Input: part model. Units: mm. Frame: model coordinates. A direction names the side the tool comes from. Give positions to 0.01 mm unless a question says otherwise; leave off trailing zeros. Loops run counter-clockwise (first coordinate to the right, second up) from the corner with the lowest first, then second, coordinate; pieces in that order, holes last. Notation, with made-up numbers: M -27.5,-17.5 L 13.5,-17.5 A34 ccw 13.5,14.5 Z; hole C -32.75,-33.75 d8. An arc over 180 degrees is marked long. One line per item, written item: value. Start each with the question number.
(1) Section A-A on z = 53.15. Output: boundary loops of the cut face in (x, y), plus the area to 3 significant figures.
(2) Pull-direction query (Y, two-part tool) for faces 1 (the cylindrical face through (-9.764, 74.362, 6.409)), 2 (the flat face through (-42.6, 3, 20)), 3 (the flat face through (-48, 3, 64.95)); classes: released by +Y, released by -Y, zero draft, split by the parting line, or undercut.
(3) Access query for faces 4 (the flat face through (-50, 32.697, 20)), 5 (the flat face through (-42.6, 3, 69)), 6 (the flat face through (-24, -8, 10)). Directions: +Z, -Z, +X, -X, +Y, -Y. A direction counts if a zero-diameter tool reaches every point of the face in a straight line with its end or side. Return the directions, or none.
(4) Pin query (flat end, axial travel): P1, Ø3, axis at y = -5.37, z = 67.95, coming from the -X side; P2, Ø1.5, axis at x = -36.5, y = 32, coming from the +Z side; P3, Ø10.5, axis at x = -52, z = 23, coming from the +Y side. Return the tip coordinate at first contact, or that it passes through.
(5) Section B-B on x = 0. Output: boundary loops of the cut face in (y, z).
(6) Section C-C on z = 38. Output: boundary loops of the cut face in (x, y), plus the area to 3 significant figures.
(7) Ray query, line 1 along Y through (x, z) = (-46.8, 67.95); line 2 along X through (y, z) = (28.5, 33); line 3 along Y through (x, z) = (-43, 18). Return the intervals inside material, ascending. Write a range as from..to.
```python
from build123d import *

# Parameters (mm, degrees)
SKETCH1_R           = 75
BASE_PLATE_DEPTH    = 15
SKETCH2_R           = 4.5
DRIVE_HOLES_DEPTH   = 10
CHAMFER1_SIZE       = 1
BASE_START          = 45
BASE_FIN_DEPTH      = 5
BASE_START_2        = 85
BASE_FIN_2_DEPTH    = 5
CUT_EXTRUDE1_REACH  = 122
CUT_EXTRUDE2_REACH  = 122
SKETCH7_R           = 1.75
BOSS_EXTRUDE1_DEPTH = 5.6
SKETCH9_R           = 1.75
CUT_EXTRUDE3_DEPTH  = 5.6
SKETCH10_W          = 4.6
SKETCH10_H          = 2.5
SKETCH10_W_2        = 6
CUT_EXTRUDE4_DEPTH  = 5.6
CUT_EXTRUDE5_DEPTH  = 2.6
BOSS_EXTRUDE2_DEPTH = 1.38
FILLET1_R           = 2
FILLET2_R           = 2
CUT_EXTRUDE6_REACH  = 37
SKETCH13_R          = 12.7
BOSS_EXTRUDE4_START = 20
BOSS_EXTRUDE4_DEPTH = 2.5
BOSS_EXTRUDE5_START = 20
BOSS_EXTRUDE5_DEPTH = 2.5
FILLET4_R           = 2


with BuildPart() as part:
    # Sketch1 → Base Plate (new body)
    with BuildSketch(Plane.XY):
        Circle(SKETCH1_R)
    extrude(amount=BASE_PLATE_DEPTH)

    # Sketch2 → Drive Holes (cut)
    with BuildSketch(Plane(origin=(0, 0, 0), x_dir=(-1, 0, 0), z_dir=(0, 0, -1))):
        with Locations((0, -25)):
            Circle(SKETCH2_R)
        with Locations((-23.776412907, -7.725424859)):
            Circle(SKETCH2_R)
        with Locations((-14.694631307, 20.225424859)):
            Circle(SKETCH2_R)
        with Locations((14.694631307, 20.225424859)):
            Circle(SKETCH2_R)
        with Locations((23.776412907, -7.725424859)):
            Circle(SKETCH2_R)
    extrude(amount=-DRIVE_HOLES_DEPTH, mode=Mode.SUBTRACT)

    # Chamfer1
    chamfer1_edges = [part.edges().sort_by_distance(p)[0] for p in [
        (28.276412907, -7.725424859, 0),
        (19.194631307, 20.225424859, 0),
        (-10.194631307, 20.225424859, 0),
        (-19.276412907, -7.725424859, 0),
        (4.5, -25, 0),
    ]]
    chamfer(chamfer1_edges, length=CHAMFER1_SIZE)

    # Sketch4 → Base Fin (add)
    with BuildSketch(Plane(origin=(0, 0, 0), x_dir=(0, 0, -1), z_dir=(1, 0, 0)).offset(BASE_START)):
        with BuildLine():
            Line((-15, 50), (-65.791986374, 16.233382914))
            ThreePointArc((-65.791986374, 16.233382914), (-74.493324261, 0), (-65.791986374, -16.233382914))
            Line((-65.791986374, -16.233382914), (-15, -50))
            Line((-15, -50), (-15, 50))
        make_face()
    extrude(amount=-BASE_FIN_DEPTH)

    # Sketch5 → Base Fin 2 (add)
    with BuildSketch(Plane.ZY.offset(-40).offset(BASE_START_2)):
        with BuildLine():
            Line((15, 50), (15, -50))
            Line((15, -50), (65.791986374, -16.233382914))
            ThreePointArc((65.791986374, -16.233382914), (74.493324261, 0), (65.791986374, 16.233382914))
            Line((65.791986374, 16.233382914), (15, 50))
        make_face()
    extrude(amount=-BASE_FIN_2_DEPTH)

    # Sketch6 → Cut-Extrude1 (cut, up to next)
    with BuildSketch(Plane.ZY.offset(45), mode=Mode.PRIVATE) as cut_extrude1_sk1:
        with BuildLine():
            Line((64, 8.832406236), (64, -9.567593764))
            ThreePointArc((64, -9.567593764), (63.487436867, -10.805030631), (62.25, -11.317593764))
            Line((62.25, -11.317593764), (24.05, -11.317593764))
            ThreePointArc((24.05, -11.317593764), (22.812563133, -10.805030631), (22.3, -9.567593764))
            Line((22.3, -9.567593764), (22.3, 8.832406236))
            ThreePointArc((22.3, 8.832406236), (22.812563133, 10.069843103), (24.05, 10.582406236))
            Line((24.05, 10.582406236), (62.25, 10.582406236))
            ThreePointArc((62.25, 10.582406236), (63.487436867, 10.069843103), (64, 8.832406236))
        make_face()
    cut_extrude1_tool1 = extrude(cut_extrude1_sk1.sketch, amount=-CUT_EXTRUDE1_REACH, mode=Mode.PRIVATE) & part.part
    add(cut_extrude1_tool1.solids().sort_by_distance((-45, -0.367594, 43.15))[0], mode=Mode.SUBTRACT)

    # Sketch7 → Cut-Extrude2 (cut, up to next)
    with BuildSketch(Plane.ZY.offset(45), mode=Mode.PRIVATE) as cut_extrude2_sk1:
        with Locations((18.35, 4.632406236)):
            Circle(SKETCH7_R)
    cut_extrude2_tool1 = extrude(cut_extrude2_sk1.sketch, amount=-CUT_EXTRUDE2_REACH, mode=Mode.PRIVATE) & part.part
    add(cut_extrude2_tool1.solids().sort_by_distance((-45, 4.632406, 18.35))[0], mode=Mode.SUBTRACT)
    # Sketch7 → Cut-Extrude2 (cut, up to next)
    with BuildSketch(Plane.ZY.offset(45), mode=Mode.PRIVATE) as cut_extrude2_sk2:
        with Locations((18.35, -5.367593764)):
            Circle(SKETCH7_R)
    cut_extrude2_tool2 = extrude(cut_extrude2_sk2.sketch, amount=-CUT_EXTRUDE2_REACH, mode=Mode.PRIVATE) & part.part
    add(cut_extrude2_tool2.solids().sort_by_distance((-45, -5.367594, 18.35))[0], mode=Mode.SUBTRACT)
    # Sketch7 → Cut-Extrude2 (cut, up to next)
    with BuildSketch(Plane.ZY.offset(45), mode=Mode.PRIVATE) as cut_extrude2_sk3:
        with Locations((67.95, -5.367593764)):
            Circle(SKETCH7_R)
    cut_extrude2_tool3 = extrude(cut_extrude2_sk3.sketch, amount=-CUT_EXTRUDE2_REACH, mode=Mode.PRIVATE) & part.part
    add(cut_extrude2_tool3.solids().sort_by_distance((-45, -5.367594, 67.95))[0], mode=Mode.SUBTRACT)
    # Sketch7 → Cut-Extrude2 (cut, up to next)
    with BuildSketch(Plane.ZY.offset(45), mode=Mode.PRIVATE) as cut_extrude2_sk4:
        with Locations((67.95, 4.632406236)):
            Circle(SKETCH7_R)
    cut_extrude2_tool4 = extrude(cut_extrude2_sk4.sketch, amount=-CUT_EXTRUDE2_REACH, mode=Mode.PRIVATE) & part.part
    add(cut_extrude2_tool4.solids().sort_by_distance((-45, 4.632406, 67.95))[0], mode=Mode.SUBTRACT)

    # Sketch8 → Boss-Extrude1 (add)
    with BuildSketch(Plane.ZY.offset(45)):
        with BuildLine():
            Line((70.95, 4.632406236), (70.95, -5.367593764))
            ThreePointArc((70.95, -5.367593764), (67.95, -8.367593764), (64.95, -5.367593764))
            Line((64.95, -5.367593764), (64.95, 4.632406236))
            ThreePointArc((64.95, 4.632406236), (67.95, 7.632406236), (70.95, 4.632406236))
        make_face()
        with BuildLine():
            Line((15, 7.632406236), (15, 0))
            Line((15, 0), (15, -8.367593764))
            Line((15, -8.367593764), (18.35, -8.367593764))
            ThreePointArc((18.35, -8.367593764), (20.471320344, -7.488914107), (21.35, -5.367593764))
            Line((21.35, -5.367593764), (21.35, 4.632406236))
            ThreePointArc((21.35, 4.632406236), (20.471320344, 6.75372658), (18.35, 7.632406236))
            Line((18.35, 7.632406236), (15, 7.632406236))
        make_face()
    extrude(amount=BOSS_EXTRUDE1_DEPTH)

    # Sketch9 → Cut-Extrude3 (cut)
    with BuildSketch(Plane(origin=(-45, 0, 0), x_dir=(0, 0, -1), z_dir=(1, 0, 0))):
        with Locations((-67.95, -5.367593764)):
            Circle(SKETCH9_R)
        with Locations((-67.95, 4.632406236)):
            Circle(SKETCH9_R)
        with Locations((-18.35, -5.367593764)):
            Circle(SKETCH9_R)
        with Locations((-18.35, 4.632406236)):
            Circle(SKETCH9_R)
    extrude(amount=-CUT_EXTRUDE3_DEPTH, mode=Mode.SUBTRACT)

    # Sketch10 → Cut-Extrude4 (cut)
    with BuildSketch(Plane.ZY.offset(50.6)):
        with Locations((19.05, -0.367593764)):
            Rectangle(SKETCH10_W, SKETCH10_H)
        with Locations((67.95, -0.324654002)):
            Rectangle(SKETCH10_W_2, SKETCH10_H)
    extrude(amount=-CUT_EXTRUDE4_DEPTH, mode=Mode.SUBTRACT)

    # Sketch11 → Cut-Extrude5 (cut)
    with BuildSketch(Plane(origin=(-40, 0, 0), x_dir=(0, 0, -1), z_dir=(1, 0, 0))):
        Polygon((-65.075, -7.027475788), (-65.075, -3.70771174), (-67.95, -2.047829716), (-70.825, -3.70771174), (-70.825, -7.027475788), (-67.95, -8.687357811), align=None)
        Polygon((-65.075, 2.972524212), (-65.075, 6.29228826), (-67.95, 7.952170284), (-70.825, 6.29228826), (-70.825, 2.972524212), (-67.95, 1.312642189), align=None)
        Polygon((-15.475, -7.027475788), (-15.475, -3.70771174), (-18.35, -2.047829716), (-21.225, -3.70771174), (-21.225, -7.027475788), (-18.35, -8.687357811), align=None)
        Polygon((-15.475, 2.972524212), (-15.475, 6.29228826), (-18.35, 7.952170284), (-21.225, 6.29228826), (-21.225, 2.972524212), (-18.35, 1.312642189), align=None)
    extrude(amount=-CUT_EXTRUDE5_DEPTH, mode=Mode.SUBTRACT)

    # Sketch12 → Boss-Extrude2 (add)
    with BuildSketch(Plane(origin=(-40, 0, 0), x_dir=(0, 0, -1), z_dir=(1, 0, 0))):
        with BuildLine():
            Line((-44.572101834, -11.317593764), (-44.572101834, 10.582406236))
            Line((-44.572101834, 10.582406236), (-24.05, 10.582406236))
            ThreePointArc((-24.05, 10.582406236), (-22.812563133, 10.069843104), (-22.3, 8.832406236))
            Line((-22.3, 8.832406236), (-22.3, -9.567593764))
            ThreePointArc((-22.3, -9.567593764), (-22.812563133, -10.805030631), (-24.05, -11.317593764))
            Line((-24.05, -11.317593764), (-44.572101834, -11.317593764))
        make_face()
    extrude(amount=-BOSS_EXTRUDE2_DEPTH)

    # Fillet1
    fillet1_edges = [part.edges().sort_by_distance(p)[0] for p in [
        (-45, -29.183796882, 15),
        (-47.8, -8.367593764, 15),
        (-47.8, 7.632406236, 15),
        (42.5, 50, 15),
        (42.5, -50, 15),
        (45, 0, 15),
        (-42.5, 50, 15),
        (-42.5, -50, 15),
        (-45, 28.816203118, 15),
    ]]
    fillet(fillet1_edges, radius=FILLET1_R)

    # Fillet2
    fillet2_edges = [part.edges().sort_by_distance(p)[0] for p in [
        (-75, 0, 15),
    ]]
    fillet(fillet2_edges, radius=FILLET2_R)

    # Sketch13 → Cut-Extrude6 (cut, up to next)
    with BuildSketch(Plane.ZY.offset(-40), mode=Mode.PRIVATE) as cut_extrude6_sk1:
        with Locations((53.15, -0.367593764)):
            Circle(SKETCH13_R)
    cut_extrude6_tool1 = extrude(cut_extrude6_sk1.sketch, amount=-CUT_EXTRUDE6_REACH, mode=Mode.PRIVATE) & part.part
    add(cut_extrude6_tool1.solids().sort_by_distance((40, -0.367594, 53.15))[0], mode=Mode.SUBTRACT)

    # Sketch17 → Boss-Extrude4 (add, symmetric)
    with BuildSketch(Plane(origin=(0, 0, 0), x_dir=(1, 0, 0), z_dir=(0, 1, 0)).offset(BOSS_EXTRUDE4_START)):
        Polygon((-42.667233731, -13), (-42.667233731, -30.724225819), (-60.39145955, -13), align=None)
    extrude(amount=BOSS_EXTRUDE4_DEPTH, both=True)

    # Sketch18 → Boss-Extrude5 (add, symmetric)
    with BuildSketch(Plane(origin=(-60.248558799, 10.197029926, -5.539416888), x_dir=(-1, 0, 0), z_dir=(0, 1, 0)).offset(BOSS_EXTRUDE5_START)):
        Polygon((-1.857099249, 20.539416888), (-15.248558799, 33.930876438), (-15.248558799, 20.539416888), align=None)
    extrude(amount=BOSS_EXTRUDE5_DEPTH, both=True)

    # Fillet4
    fillet4_edges = [part.edges().sort_by_distance(p)[0] for p in [
        (-45.585786438, 17.5, 15.585786438),
        (-45.585786438, 22.5, 15.585786438),
        (-45, 20, 28.39145955),
        (-58.39145955, 20, 15),
        (-52.695729775, 22.5, 15),
        (-45, 22.5, 22.695729775),
        (-52.695729775, 17.5, 15),
        (-45, 17.5, 22.695729775),
        (-45.585786438, 27.697029926, 15.585786438),
        (-45.585786438, 32.697029926, 15.585786438),
        (-52.695729775, 27.697029926, 15),
        (-45, 32.697029926, 22.695729775),
        (-52.695729775, 32.697029926, 15),
        (-58.39145955, 30.197029926, 15),
        (-45, 30.197029926, 28.39145955),
        (-45, 27.697029926, 22.695729775),
    ]]
    fillet(fillet4_edges, radius=FILLET4_R)


solid = part.part
```
Output values:
1. outline: M -45,-24.64 L -40,-24.64 L -40,-11.32 L -45,-11.32 Z; M -45,10.58 L -40,10.58 L -40,24.64 L -45,24.64 Z; M 40,-24.64 L 45,-24.64 L 45,-13.07 L 40,-13.07 Z; M 40,12.33 L 45,12.33 L 45,24.64 L 40,24.64 Z
1. area: 256 mm²
2. face 1: split by the parting line
2. face 2: undercut
2. face 3: zero draft
3. face 4: +Z, -X, +Y
3. face 5: none
3. face 6: -Z
4. P1: stops at x = 40
4. P2: stops at z = 15
4. P3: stops at y = 32.71
5. outline: M -75,0 L -30.5,0 L -29.5,1 L -29.5,10 L -20.5,10 L -20.5,1 L -19.5,0 L 75,0 L 75,13 A2 ccw 73,15 L -73,15 A2 ccw -75,13 Z
6. outline: M -45,-34.71 L -40,-34.71 L -40,34.71 L -45,34.71 L -45,10.58 L -41.38,10.58 L -41.38,-11.32 L -45,-11.32 Z; M 40,-34.71 L 45,-34.71 L 45,34.71 L 40,34.71 Z
6. area: 615 mm²
7. line 1: y = -8.37..-7.12, -3.62..-1.57, 0.93..2.88, 6.38..7.63
7. line 2: x = -45..-40, 40..45
7. line 3: y = -48.01..-7.08, -3.65..2.92, 6.35..48.01
